Model file for the job. Use its own axes, mm. Face numbers are marked on the shaded views. A direction names the side the tool comes from. Round coordinates to 2 decimals unless told otherwise and drop trailing zeros. Order: outer loops, then holes, each group sorted by start corner. A loop starts at its lowest first (then second) coordinate and runs counter-clockwise, first axis right, second up. Notation, with made-up numbers: M 6.25,83 L 60.25,83 A31 cw 60.25,108 Z; hole C 28,-34 d5. An arc over 180 degrees is marked long. Return JSON: item names as keys, results as strings. Group by question number.
Item 1: Pin check, flat tips, straight feed: pin 1 Ø0.6 at (y, z) = (-1.5, 0.5) entering from -X; pin 2 Ø2 at (x, z) = (-5, -2) entering from -Y; pin 3 Ø1.5 at (x, y) = (10.5, 0) entering from +Z; pin 4 Ø1 at (x, z) = (11, 1) entering from +Y. Stop position of each tip, or through.
Item 2: Probe line 1 along Y through (x, z) = (10, 0.25); line 2 along Y through (x, z) = (-5.5, 0); line 3 along Z through (x, y) = (12.45, 0). List the from-to ranges inside material, lowest first.
Item 3: Slice it at C-C on y = -0.75. Give the number of separate pieces and of enclosed holes in the cut face, then the cut area to 3 significant figures.
Item 4: Slice it at D-D on y = 2.5. Write the cut outline in (x, z), then the cut area to 3 significant figures.
Item 5: Which spindle directions (+Z, -Z, +X, -X, +Y, -Y) get a long thin tool onto all of the face, cutting with end or side? Do the marked faces 4 and 5. Say none if no direction does.
Item 6: Slice it at A-A on x = 10. Write the cut outline in (y, z).
Item 7: Pull direction Z, two halves, no side cores. Call the marked faces 1, 2 and 3: pulls with the +Z half, pulls with the -Z half, needs draft (parallel to the pull), parting line crosses it, or undercut.
Autodesk Inventor part; units mm, degrees
ref_plane "YZ Plane" through (0, 0, 0) normal (1, 0, 0) x (0, 1, 0)
ref_plane "XZ Plane" through (0, 0, 0) normal (0, 1, 0) x (-1, 0, 0)
ref_plane "XY Plane" through (0, 0, 0) normal (0, 0, 1) x (1, 0, 0)
sketch "Sketch1" plane through (0, 0, 0) normal (0, 0, 1) x (1, 0, 0)
  circle A0 centre (-10, 0) radius 1
  circle A1 centre (10, 0) radius 1
  circle A2 centre (-10, 0) radius 4
  circle A3 centre (10, 0) radius 4
  point P0 (0, 0)
  dimension "d0" = 2
  dimension "d1" = 2
  dimension "d3" = 20
  dimension "d4" = 10
  dimension "d5" = 8
  dimension "d6" = 8
extrude "Extrusion1" add sketch "Sketch1" against normal mid plane 18
sketch "Sketch2" plane through (0, 0, 0) normal (0, 0, 1) x (1, 0, 0)
  circle A0 centre (-10, 0) radius 4
  circle A1 centre (-10, 0) radius 1
  point P0 (0, 0)
extrude "Extrusion2" cut sketch "Sketch2" against normal mid plane 9
sketch "Sketch3" plane through (-10, 0, -4.5) normal (0, 0, 1) x (1, 0, 0)
  circle A0 centre (20, 0) radius 4
  circle A1 centre (20, 0) radius 4
  circle A2 centre (20, 0) radius 1
  point P0 (10, 0)
extrude "Extrusion3" cut sketch "Sketch3" against normal blind 4.5
mirror "Mirror1" about plane through (0, 0, 0) normal (0, 0, 1) of "Extrusion3"
sketch "Sketch6" plane through (0, 0, 0) normal (0, 1, 0) x (-1, 0, 0)
  line L0 (-6, -4.5) -> (-9, -4.5) construction
  line L1 (-9, -4.5) -> (-9, 4.5) construction
  line L2 (-9, 4.5) -> (-6, 4.5) construction
  line L3 (-6, 4.5) -> (-6, -4.5) construction
  line L4 (-11, -4.5) -> (-14, -4.5) construction
  line L5 (-14, -4.5) -> (-14, 4.5) construction
  line L6 (-14, 4.5) -> (-11, 4.5) construction
  line L7 (-11, 4.5) -> (-11, -4.5) construction
  line L8 (6, 9) -> (9, 9) construction
  line L9 (9, 9) -> (9, 4.5) construction
  line L10 (9, 4.5) -> (6, 4.5) construction
  line L11 (6, 4.5) -> (6, 9) construction
  line L12 (11, 9) -> (14, 9) construction
  line L13 (14, 9) -> (14, 4.5) construction
  line L14 (14, 4.5) -> (11, 4.5) construction
  line L15 (11, 4.5) -> (11, 9) construction
  line L16 (14, -9) -> (11, -9) construction
  line L17 (11, -9) -> (11, -4.5) construction
  line L18 (11, -4.5) -> (14, -4.5) construction
  line L19 (14, -4.5) -> (14, -9) construction
  line L20 (9, -9) -> (6, -9) construction
  line L21 (6, -9) -> (6, -4.5) construction
  line L22 (6, -4.5) -> (9, -4.5) construction
  line L23 (9, -4.5) -> (9, -9) construction
  line L24 (6, -9) -> (14, -9) construction
  line L25 (6, -9) -> (3, -9)
  line L26 (3, -9) -> (3, -2)
  line L27 (3, -2) -> (-6, -2)
  line L28 (-6, 4.5) -> (-6, -4.5) construction
  line L29 (-6, 2) -> (3, 2)
  line L30 (3, 2) -> (3, 9)
  line L31 (3, 9) -> (6, 9)
  line L32 (6, -4.5) -> (14, -4.5) construction
  line L33 (6, -4.5) -> (6, 4.5)
  line L34 (-6, -2) -> (-9, -2)
  line L35 (-9, -4.5) -> (-9, 4.5)
  line L36 (-6, 2) -> (-9, 2)
  line L37 (6, -9) -> (9, -9)
  line L38 (9, -4.5) -> (6, -4.5)
  line L39 (11, -4.5) -> (9, -4.5)
  line L40 (9, -4.5) -> (9, -9)
  line L41 (9, -9) -> (9, -4.5)
  line L42 (9, 4.5) -> (11, 4.5)
  line L43 (14, 4.5) -> (6, 4.5)
  line L44 (9, 4.5) -> (6, 4.5)
  line L45 (9, 9) -> (11, 9)
  line L46 (9, 4.5) -> (9, 9)
  line L47 (14, 9) -> (6, 9)
  line L48 (9, 9) -> (6, 9)
  point P0 (0, 0)
  dimension "d16" = 3
  dimension "d17" = 4
  dimension "d18" = 2
extrude "Extrusion4" add sketch "Sketch6" against normal mid plane 4
sketch "Sketch7" plane through (-6, -2, -4.5) normal (-1, 0, 0) x (0, 0, 1)
  circle A0 centre (4.5, 2) radius 1
  dimension "d21" = 2
extrude "Extrusion5" cut sketch "Sketch7" against normal blind 20
chamfer "Chamfer1" distance 1 angle 45 1 edges at (-6, 0, -1)
fillet "Fillet1" radius 2 4 edges at (1.7679, 2, 2) (1.7679, 2, -2) (1.7679, -2, -2) (1.7679, -2, 2)
sketch "Sketch9" plane through (0, 0, 9) normal (0, 0, 1) x (1, 0, 0)
  circle A0 centre (-10, 0) radius 1
  circle A1 centre (-10, 0) radius 0.9
  point P0 (0, 0)
  dimension "d29" = 1.8
extrude "TREAD" add sketch "Sketch9" against normal up to surface (4.5 mm away)
sketch "Sketch11" plane through (10, 0, 4.5) normal (0, 0, 1) x (1, 0, 0)
  circle A0 centre (0, 0) radius 4
  circle A1 centre (0, 0) radius 1
  point P0 (-10, 0)
extrude "thin" cut sketch "Sketch11" against normal blind 0.1
mirror "Mirror2" about plane through (0, 0, 0) normal (0, 0, 1) of "thin"
sketch "Sketch12" plane through (10, 0, 4.4) normal (0, 0, 1) x (1, 0, 0)
  circle A0 centre (0, 0) radius 1 construction
  circle A1 centre (0, 0) radius 1.1
  point P0 (-10, 0)
  dimension "d34" = 2.2
extrude "Extrusion8" cut sketch "Sketch12" against normal up to surface (8.8 mm away)
sketch "Sketch13" plane through (0, 0, 9) normal (0, 0, 1) x (1, 0, 0)
  circle A0 centre (-10, 0) radius 0.9
  arc A1 (-6.5359, 2) -> (-6.5359, -2) centre (-10, 0) ccw
  line L0 (-3, -2) -> (-6.5359, -2)
  line L1 (-3, -2) -> (-3, 2)
  line L2 (-6.5359, 2) -> (-3, 2)
  point P0 (0, 0)
extrude "Extrusion9" cut sketch "Sketch13" against normal through all
sketch "Sketch14" plane through (-3, 0, 0) normal (-1, 0, 0) x (0, 0, 1)
  circle A0 centre (0, 0) radius 2
  circle A1 centre (0, 0) radius 1
extrude "Extrusion10" add sketch "Sketch14" along normal blind 10
chamfer "Chamfer2" distance 1 angle 45 1 edges at (-13, 0, -1)
equation "\"d6\" = d5"
properties part number "Tolerenced_Phalalnge_20_TIPmm"
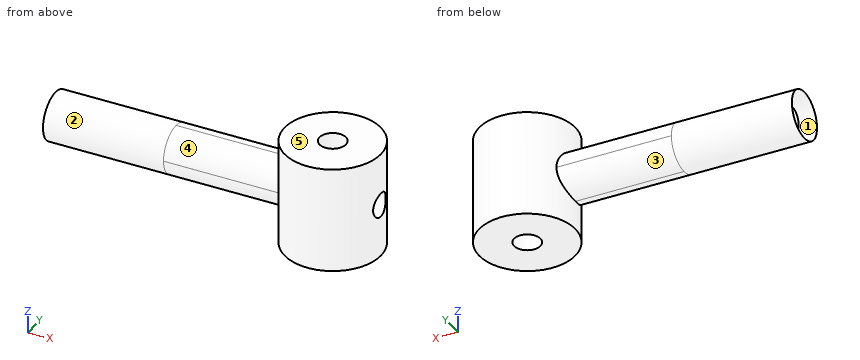
Output values:
{
 "1": {"pin 1": "x = -12.88", "pin 2": "y = -1.73", "pin 3": "z = 4.4", "pin 4": "y = 3.97"},
 "2": {"line 1": "-4 to -1.1, 1.1 to 4", "line 2": "-2 to -1, 1 to 2", "line 3": "-4.4 to -1, 1 to 4.4"},
 "3": {"separate pieces": "4", "enclosed holes": "0", "area": "91.0 mm²"},
 "4": {"outline": "M 6.88,-4.4 L 13.12,-4.4 L 13.12,4.4 L 6.88,4.4 Z", "area": "55.0 mm²"},
 "5": {"face 4": "+Z, -X, -Y", "face 5": "+Z, +X, -X, +Y, -Y"},
 "6": {"outline": "M -4,-4.4 L -1.1,-4.4 L -1.1,4.4 L -4,4.4 Z; M 1.1,-4.4 L 4,-4.4 L 4,4.4 L 1.1,4.4 Z"},
 "7": {"face 1": "undercut", "face 2": "parting line crosses it", "face 3": "pulls with the -Z half"}
}
